Here's how the part is built. I have some questions about the finished solid (model axes, mm). A direction names the side the tool comes from. Round coordinates to 2 decimals unless told otherwise and drop trailing zeros. Order: outer loops, then holes, each group sorted by start corner. A loop starts at its lowest first (then second) coordinate and runs counter-clockwise, first axis right, second up.
```python
from build123d import *

# Parameters (mm, degrees)
SKETCH1_W                       = 50
SKETCH1_H                       = 30
SKETCH1_R                       = 1.65
SKETCH1_R_2                     = 11
BOSS_EXTRUDE1_DEPTH             = 36
TAP_DRILL_FOR_M4X0_7_TAP1_D     = 3.3
TAP_DRILL_FOR_M4X0_7_TAP1_DEPTH = 10
TAP_DRILL_FOR_M4X0_7_TAP1_TIP   = 0.991420021
TAP_DRILL_FOR_M4X0_7_TAP2_D     = 3.3
TAP_DRILL_FOR_M4X0_7_TAP2_DEPTH = 13
TAP_DRILL_FOR_M4X0_7_TAP2_TIP   = 0.991420021
CHAMFER1_SIZE                   = 0.5


with BuildPart() as part:
    # Sketch1 → Boss-Extrude1 (new body)
    # profile 1 of 7: a face of its own
    with BuildSketch(Plane(origin=(0, 0, 0), x_dir=(1, 0, 0), z_dir=(0, 1, 0))):
        with Locations((25, 15)):
            Rectangle(SKETCH1_W, SKETCH1_H)
        with Locations((36.366741508, 3.633258492)):
            Circle(SKETCH1_R, mode=Mode.SUBTRACT)
        with Locations((13.633258492, 3.633258492)):
            Circle(SKETCH1_R, mode=Mode.SUBTRACT)
        with Locations((8.925, 15)):
            Circle(SKETCH1_R, mode=Mode.SUBTRACT)
        with Locations((13.633258492, 26.366741508)):
            Circle(SKETCH1_R, mode=Mode.SUBTRACT)
        with Locations((36.366741508, 26.366741508)):
            Circle(SKETCH1_R, mode=Mode.SUBTRACT)
        with Locations((41.075, 15)):
            Circle(SKETCH1_R, mode=Mode.SUBTRACT)
        with Locations(Location((25, 15, 0), (0, 0, 270))):
            Circle(SKETCH1_R_2, mode=Mode.SUBTRACT)
    # profile 2 of 7: a face of its own
    with BuildSketch(Plane(origin=(0, 0, 0), x_dir=(1, 0, 0), z_dir=(0, 1, 0))):
        with Locations((41.075, 15)):
            Circle(SKETCH1_R)
    # profile 3 of 7: a face of its own
    with BuildSketch(Plane(origin=(0, 0, 0), x_dir=(1, 0, 0), z_dir=(0, 1, 0))):
        with Locations((36.366741508, 26.366741508)):
            Circle(SKETCH1_R)
    # profile 4 of 7: a face of its own
    with BuildSketch(Plane(origin=(0, 0, 0), x_dir=(1, 0, 0), z_dir=(0, 1, 0))):
        with Locations((36.366741508, 3.633258492)):
            Circle(SKETCH1_R)
    # profile 5 of 7: a face of its own
    with BuildSketch(Plane(origin=(0, 0, 0), x_dir=(1, 0, 0), z_dir=(0, 1, 0))):
        with Locations((13.633258492, 3.633258492)):
            Circle(SKETCH1_R)
    # profile 6 of 7: a face of its own
    with BuildSketch(Plane(origin=(0, 0, 0), x_dir=(1, 0, 0), z_dir=(0, 1, 0))):
        with Locations((8.925, 15)):
            Circle(SKETCH1_R)
    # profile 7 of 7: a face of its own
    with BuildSketch(Plane(origin=(0, 0, 0), x_dir=(1, 0, 0), z_dir=(0, 1, 0))):
        with Locations((13.633258492, 26.366741508)):
            Circle(SKETCH1_R)
    extrude(amount=-BOSS_EXTRUDE1_DEPTH)

    # Tap Drill for M4x0.7 Tap1
    with Locations(Plane(origin=(8.925, 0, -15), x_dir=(0, 0, 1), z_dir=(0, 1, 0))):
        with Locations((0, 0), (-11.366741508, 4.708258492), (-11.366741508, 27.441741508), (0, 32.15), (11.366741508, 27.441741508), (11.366741508, 4.708258492)):
            Hole(TAP_DRILL_FOR_M4X0_7_TAP1_D / 2, depth=TAP_DRILL_FOR_M4X0_7_TAP1_DEPTH)
            with Locations((0, 0, -(TAP_DRILL_FOR_M4X0_7_TAP1_DEPTH + TAP_DRILL_FOR_M4X0_7_TAP1_TIP / 2))):  # 118° drill point
                Cone(0, TAP_DRILL_FOR_M4X0_7_TAP1_D / 2, TAP_DRILL_FOR_M4X0_7_TAP1_TIP, mode=Mode.SUBTRACT)

    # Tap Drill for M4x0.7 Tap2
    with Locations(Plane(origin=(7.45, -5.9, 0), x_dir=(1, 0, 0), z_dir=(0, 0, 1))):
        with Locations((0, 0), (35.1, 0), (35.1, -24.2), (0, -24.2)):
            Hole(TAP_DRILL_FOR_M4X0_7_TAP2_D / 2, depth=TAP_DRILL_FOR_M4X0_7_TAP2_DEPTH)
            with Locations((0, 0, -(TAP_DRILL_FOR_M4X0_7_TAP2_DEPTH + TAP_DRILL_FOR_M4X0_7_TAP2_TIP / 2))):  # 118° drill point
                Cone(0, TAP_DRILL_FOR_M4X0_7_TAP2_D / 2, TAP_DRILL_FOR_M4X0_7_TAP2_TIP, mode=Mode.SUBTRACT)

    # Chamfer1
    chamfer1_edges = [part.edges().sort_by_distance(p)[0] for p in [
        (0, -18, 0),
        (0, -18, -30),
        (50, -18, -30),
        (25, -36, 0),
        (50, -18, 0),
        (50, -36, -15),
        (13.633258492, 0, -1.983258492),
        (25, -36, -30),
        (36.366741508, 0, -1.983258492),
        (0, -36, -15),
        (41.075, 0, -13.35),
        (36.366741508, 0, -24.716741508),
        (13.633258492, 0, -24.716741508),
        (8.925, 0, -13.35),
        (9.1, -30.1, 0),
        (44.2, -30.1, 0),
        (44.2, -5.9, 0),
        (25, -36, -26),
        (9.1, -5.9, 0),
        (0, 0, -15),
        (25, 0, -30),
        (50, 0, -15),
        (25, 0, 0),
        (25, 0, -26),
    ]]
    chamfer(chamfer1_edges, length=CHAMFER1_SIZE)


solid = part.part
```
1. If we section it at A-A, the plane y = -20.5: Write out the boundary of the cut face in (x, z).
Evaluation:
outline: (0, -29.5) - (0.5, -30) - (49.5, -30) - (50, -29.5) - (50, -0.5) - (49.5, 0) - (0.5, 0) - (0, -0.5) - close; hole circle Ø22 at (25, -15)
2. If we mould it in two halves opening along Y, with no side actions, what happens to faces 1 (the conical face through (7.41, -29.82, -13.82)), 2 (the conical face through (36.113, -10.819, -3.501)), 3 (the conical face through (42.82, -30.01, -13.82)), 4 (the cylindrical face through (15.27, -5.32, -3.42))? For each: released by +Y, released by -Y, zero draft, split by the parting line, or undercut.
Evaluation:
face 1: undercut
face 2: released by +Y
face 3: undercut
face 4: zero draft
3. I'm going to push flat-ended pins straight in: P1, Ø2.5, axis at x = 36.37, z = -26.37, coming from the +Y side; P2, Ø2.5, axis at x = 42.55, y = -30.1, coming from the +Z side; P3, Ø17.5, axis at x = 25, z = -15, coming from the +Y side. Where does each tip first touch, or does it pass through?
Evaluation:
P1: stops at y = -10.24
P2: stops at z = -13.24
P3: passes through
4. If we section it at B-B, the plane z = -10: State how many separate pieces and enclosed holes the cut face has, and give its area (3 significant figures).
Evaluation:
separate pieces: 2
enclosed holes: 4
area: 1,060 mm2
5. On a 3-axis mill with a long thin cutter (end or side, diameter ignored), from which of +Z, -Z, +X, -X, +Y, -Y can I reach the whole of each face in a straight line? I mean faces 5 (the cylindrical face through (37.76, -5.32, -4.52)), 6 (the flat face through (50, -18, -15)). Say none if no direction works.
Evaluation:
face 5: +Y
face 6: +Z, -Z, +X, +Y, -Y
6. I need wall thicknesses on probe 1 along X at (y, z) = (-7.5, -15) (3 decimals); probe 2 along X at (y, z) = (-15.5, -15.25); probe 3 along Y at (x, z) = (7, -7.5). Which ranges of each line are inside material? Lowest first, please.
Evaluation:
probe 1: x = 0 to 7.275, 10.575 to 14, 36 to 39.425, 42.725 to 50
probe 2: x = 0 to 14, 36 to 50
probe 3: y = -36 to -31.69, -28.51 to -7.49, -4.31 to 0
